Can you work these out from the model? Positions are in its coordinate system, mm. A direction names the side the tool comes from. Give positions to 0.01 mm unless a question says otherwise; leave off trailing zeros. Order: outer loops, then holes, each group sorted by start corner. A loop starts at its lowest first (then second) coordinate and runs counter-clockwise, first axis right, second up. Notation, with made-up numbers: (7.5, -7.75) - (45.5, -7.75) arc R20 ccw to (45.5, 17.25) - close; hole circle Ø5 at (73, 24.5). An arc over 180 degrees is marked (long way). Use one line per item in the form item = value. Start each with the question number.
1) Suppose I cut it at C-C, the plane y = -60.5. Write out the boundary of the cut face in (x, z).
2) Suppose I cut it at D-D, the plane z = 39. Write out the boundary of the cut face in (x, y).
3) Suppose I cut it at B-B, the plane x = -52. Write out the boundary of the cut face in (y, z).
4) For pin 1 (4 mm diameter, centred on y = -63, z = 4, fed in from -X); pin 2 (23 mm diameter, centred on y = -22, z = 48.5, fed in from +X); pin 3 (20.5 mm diameter, centred on x = -51.5, y = 17.5, fed in from -Z); pin 4 (3 mm diameter, centred on y = -41, z = 24, fed in from -X), each with a flat end and sliding along its axis, tell me the tip position at first contact or that it passes through.
5) Please list where these lines run through material, in increasing order: probe 1 along Y at (x, z) = (-41, 53); probe 2 along Y at (x, z) = (-50, 14.5); probe 3 along Z at (x, y) = (-41.5, -6).
6) Which directions (+Z, -Z, +X, -X, +Y, -Y) give clear straight access to the entire face, cutting with the end or side of a thin tool? Please do faces 1 (the flat face through (-49, 13, 14.779)), 2 (the flat face through (-69.493, -5, 37)), 3 (the flat face through (-49, 0, 21)), 4 (the flat face through (-49, -50.8, 51)), 5 (the flat face through (-28.549, -5, 37)).
7) Suppose I cut it at A-A, the plane z = 51.5. Write out the boundary of the cut face in (x, y), and give its area (3 significant figures).
8) We'd pull the mould along Y, two halves only. Please class faces 6 (the flat face through (-65.27, -63.32, 20.08)), 7 (the flat face through (-49, -76.2, 29)), 8 (the flat face through (-49, -25, 48.059)): released by +Y, released by -Y, zero draft, split by the parting line, or undercut.
```python
from build123d import *

# Parameters (mm, degrees)
F0_W     = 40.943392
F0_H     = 21.0566
F1_DEPTH = 50.8
F3_DEPTH = 25.4
F4_W     = 40.943392
F4_H     = 45.667097
F5_DEPTH = 25.4


with BuildPart() as f1:
    # F0 (on Front) → F1 (new body)
    with BuildSketch(Plane.XZ):
        with Locations((-49.021153, 37.531126)):
            Rectangle(F0_W, F0_H)
    extrude(amount=F1_DEPTH)

    # F2 (on face) → F3 (join)
    with BuildSketch(Plane.XZ.offset(50.8)):
        Polygon((-16.144358, 58.535154), (-81.071265, 58.869848), (-49.021153, -19.816248), align=None)
    extrude(amount=F3_DEPTH)

    # F4 (on face) → F5 (join)
    with BuildSketch(Plane(origin=(0, 0, 0), x_dir=(-1, 0, 0), z_dir=(0, 1, 0))):
        with Locations((49.021153, 37.612088)):
            Rectangle(F4_W, F4_H)
    extrude(amount=F5_DEPTH)


solid = f1.part
```
Result sheet:
q1.outline = (-81.07, 58.87) - (-49.02, -19.82) - (-16.14, 58.54) - close
q2.outline = (-72.98, -76.2) - (-24.34, -76.2) - (-24.34, -50.8) - (-28.55, -50.8) - (-28.55, 25.4) - (-69.49, 25.4) - (-69.49, -50.8) - (-72.98, -50.8) - close
q3.outline = (-76.2, -12.5) - (-50.8, -12.5) - (-50.8, 27) - (0, 27) - (0, 14.78) - (25.4, 14.78) - (25.4, 60.45) - (0, 60.45) - (0, 48.06) - (-50.8, 48.06) - (-50.8, 58.72) - (-76.2, 58.72) - close
q4.pin_1 = -59.54
q4.pin_2 = -28.55
q4.pin_3 = 14.78
q4.pin_4 = through
q5.probe_1 = -76.2 to -50.8, 0 to 25.4
q5.probe_2 = -76.2 to -50.8
q5.probe_3 = 27 to 48.06
q6.face_1 = -Z, +X, -X, +Y
q6.face_2 = +Z, -Z, -X, +Y
q6.face_3 = -Z, +X, -X
q6.face_4 = +Z
q6.face_5 = +Z, -Z, +X, +Y
q7.outline = (-78.07, -76.2) - (-19.1, -76.2) - (-19.1, -50.8) - (-78.07, -50.8) - close; (-69.49, 0) - (-28.55, 0) - (-28.55, 25.4) - (-69.49, 25.4) - close
q7.area = 2,540 mm²
q8.face_6 = zero draft
q8.face_7 = released by -Y
q8.face_8 = undercut
